Input: part model. Units: mm. Frame: model coordinates. A direction names the side the tool comes from. Give positions to 0.01 mm unless a question says otherwise; leave off trailing zeros. Write each loop counter-clockwise with the first axis right and the second up, starting at its lowest first coordinate (ties: lowest second). Pieces come first, ordered by that corner, then holes. Notation, with made-up numbers: (51.25, -33) -> (86.25, -33) arc R8 cw to (86.25, -18) -> close; hole circle Ø4 at (55, 80.25). An arc over 180 degrees is marked (long way). Return JSON: item names as keys, results as strings. Group by question number.
Item 1: Section B-B, the plane y = 1.25. Return loops of the section in (x, z), then the cut area to 3 significant figures.
Item 2: Mould query, pull axis X, two halves, no side actions, for faces 1 (the face through (-3.226, -11.456, -7.007)), 2 (the face through (10, -5, -0.5)), 3 (the face through (9.7, -0.7, -6.3)), 4 (the face through (0, 7.4, -7)). Classes: released by +X, released by -X, zero draft, split by the parting line, or undercut.
Item 3: Section A-A, the plane x = -8. Return loops of the section in (y, z).
Item 4: Section C-C, the plane z = -4.75. Return loops of the section in (x, y), then the cut area to 3 significant figures.
Item 5: Pin query (flat end, axial travel): P1, Ø2, axis at x = 4, y = 5, coming from the +Z side; P2, Ø1.5, axis at x = -10, z = -3.5, coming from the -Y side; P3, Ø4, axis at y = -8, z = -3, coming from the -X side. Return the tip coordinate at first contact, or that it passes through.
Item 6: Section D-D, the plane x = -3.5. Return loops of the section in (y, z).
Item 7: Line query: line 1 (Y direction, x = 13.5, z = -2.25); line 2 (Y direction, x = 12.5, z = -6.6); line 3 (Z direction, x = -15.5, y = -4.5). Output: solid intervals per line, ascending. Write a range as [from, to].
Item 8: Set-up query: faces 5 (the face through (-14, 2.7, -3)), 6 (the face through (4.786, -1.051, 2.632)), 7 (the face through (14, -2.7, -3)). Return all of +Z, -Z, +X, -X, +Y, -Y with unobstructed straight access to the full face (end or side cutting, diameter ignored); none if empty.
from build123d import *

# Parameters (mm, degrees)
P_IDAT_VYSUNUT_M1_DEPTH  = 1.4
P_IDAT_VYSUNUT_M2_DEPTH  = 2.5
SKICA3_R                 = 2.7
ODEBRAT_VYSUNUT_M1_DEPTH = 2.5
P_IDAT_VYSUNUT_M3_DEPTH  = 7.5
ODEBRAT_START            = -7.5
ODEBRAT_VYSUNUT_M2_DEPTH = 7.5
SKICA9_W                 = 31.786483692
SKICA9_H                 = 14.8
P_IDAT_VYSUNUT_M5_DEPTH  = 1
SKICA6_R                 = 3.25
ODEBRAT_VYSUNUT_M3_DEPTH = 1.2
SKICA7_R                 = 0.95
ODEBRAT_VYSUNUT_M5_DEPTH = 7
P_IDAT_VYSUNUT_M7_DEPTH  = 1


with BuildPart() as part:
    # Skica1 → Přidat vysunutím1 (new body)
    with BuildSketch(Plane.XY):
        with BuildLine():
            ThreePointArc((-17.587282337, 6.5), (-18.735542789, 0.736163289), (-18.043073463, -5.1))
            Line((-18.043073463, -5.1), (-15.043073463, -5.1))
            Line((-15.043073463, -5.1), (-15.043073463, -6.5))
            Line((-15.043073463, -6.5), (17.587282337, -6.5))
            ThreePointArc((17.587282337, -6.5), (18.735542789, -0.736163289), (18.043073463, 5.1))
            Line((18.043073463, 5.1), (15.043073463, 5.1))
            Line((15.043073463, 5.1), (15.043073463, 6.5))
            Line((15.043073463, 6.5), (-17.587282337, 6.5))
        make_face()
    extrude(amount=P_IDAT_VYSUNUT_M1_DEPTH)

    # Skica2 → Přidat vysunutím2 (add)
    with BuildSketch(Plane.XY.offset(1.4)):
        with BuildLine():
            ThreePointArc((-4.9, 0), (4.82555799, -0.850876071), (-4.604493842, 1.675898702))
            Line((-4.604493842, 1.675898702), (-6.577848346, 2.394141003))
            ThreePointArc((-6.577848346, 2.394141003), (-6.893654271, 1.215537244), (-7, 0))
            Line((-7, 0), (-4.9, 0))
        make_face()
    extrude(amount=P_IDAT_VYSUNUT_M2_DEPTH)

    # Skica3 → Odebrat vysunutím1 (cut)
    with BuildSketch(Plane.XY.offset(1.4)):
        with Locations((-12.5, 0)):
            Circle(SKICA3_R)
        with Locations((12.5, 0)):
            Circle(SKICA3_R)
    extrude(amount=-ODEBRAT_VYSUNUT_M1_DEPTH, mode=Mode.SUBTRACT)

    # Skica4 → Přidat vysunutím3 (add)
    with BuildSketch(Plane(origin=(0, 0, 0), x_dir=(-1, 0, 0), z_dir=(0, 0, -1))):
        with BuildLine():
            Line((14.493241846, 6.5), (-14.493241846, 6.5))
            ThreePointArc((-14.493241846, 6.5), (-15.192361337, 4.636401214), (-15.652924941, 2.7))
            Line((-15.652924941, 2.7), (-12.5, 2.7))
            ThreePointArc((-12.5, 2.7), (-10.590811691, 1.909188309), (-9.8, 0))
            ThreePointArc((-9.8, 0), (-10.590811691, -1.909188309), (-12.5, -2.7))
            Line((-12.5, -2.7), (-15.652924941, -2.7))
            ThreePointArc((-15.652924941, -2.7), (-15.192361337, -4.636401214), (-14.493241846, -6.5))
            Line((-14.493241846, -6.5), (14.493241846, -6.5))
            ThreePointArc((14.493241846, -6.5), (15.192361337, -4.636401214), (15.652924941, -2.7))
            Line((15.652924941, -2.7), (12.5, -2.7))
            ThreePointArc((12.5, -2.7), (9.8, 0), (12.5, 2.7))
            Line((12.5, 2.7), (15.652924941, 2.7))
            ThreePointArc((15.652924941, 2.7), (15.192361337, 4.636401214), (14.493241846, 6.5))
        make_face()
    extrude(amount=P_IDAT_VYSUNUT_M3_DEPTH)

    # Skica5 → Odebrat vysunutím2 (cut)
    with BuildSketch(Plane(origin=(0, 0, 0), x_dir=(-1, 0, 0), z_dir=(0, 0, -1)).offset(ODEBRAT_START)):
        with BuildLine():
            Line((15.043073463, -6.5), (15.043073463, -5.1))
            ThreePointArc((15.043073463, -5.1), (14.784738094, -5.80651175), (14.493241846, -6.5))
            Line((14.493241846, -6.5), (15.043073463, -6.5))
        make_face()
        with BuildLine():
            ThreePointArc((-15.043073463, 5.1), (-14.784738094, 5.80651175), (-14.493241846, 6.5))
            Line((-14.493241846, 6.5), (-15.043073463, 6.5))
            Line((-15.043073463, 6.5), (-15.043073463, 5.1))
        make_face()
    extrude(amount=ODEBRAT_VYSUNUT_M2_DEPTH, mode=Mode.SUBTRACT)

    # Skica9 → Přidat vysunutím5 (add)
    with BuildSketch(Plane(origin=(0, 0, -7.5), x_dir=(-1, 0, 0), z_dir=(0, 0, -1))):
        Rectangle(SKICA9_W, SKICA9_H)
    extrude(amount=-P_IDAT_VYSUNUT_M5_DEPTH)

    # Skica6 → Odebrat vysunutím3 (cut)
    with BuildSketch(Plane(origin=(0, 0, -7.5), x_dir=(-1, 0, 0), z_dir=(0, 0, -1))):
        with Locations((-12.5, 0)):
            Circle(SKICA6_R)
        with Locations((12.5, 0)):
            Circle(SKICA6_R)
    extrude(amount=-ODEBRAT_VYSUNUT_M3_DEPTH, mode=Mode.SUBTRACT)

    # Skica7 → Odebrat vysunutím5 (cut)
    with BuildSketch(Plane(origin=(0, 0, -7.5), x_dir=(-1, 0, 0), z_dir=(0, 0, -1))):
        with Locations((10.083296, 4.829031143)):
            Circle(SKICA7_R)
        with Locations((-10.083296, -4.829031143)):
            Circle(SKICA7_R)
    extrude(amount=-ODEBRAT_VYSUNUT_M5_DEPTH, mode=Mode.SUBTRACT)

    # Skica12 → Přidat vysunutím7 (add)
    with BuildSketch(Plane(origin=(0, 0, -7.5), x_dir=(-1, 0, 0), z_dir=(0, 0, -1))):
        Polygon((-5, -7.4), (-1.5, -15.4), (1.5, -15.4), (5, -7.4), align=None)
    extrude(amount=-P_IDAT_VYSUNUT_M7_DEPTH)


solid = part.part
Answer below:
{
 "1": {"outline": "(-18.71, 0) -> (-14.89, 0) -> (-14.89, 1.4) -> (-18.71, 1.4) -> close; (-15.89, -7.5) -> (-15.5, -7.5) -> (-15.5, -6.5) -> (-15.89, -6.5) -> close; (-10.11, -6.3) -> (-9.5, -6.3) -> (-9.5, -7.5) -> (9.5, -7.5) -> (9.5, -6.3) -> (10.11, -6.3) -> (10.11, 1.4) -> (4.74, 1.4) -> (4.74, 3.9) -> (-6.89, 3.9) -> (-6.89, 1.4) -> (-10.11, 1.4) -> close; (14.89, 0) -> (18.71, 0) -> (18.71, 1.4) -> (14.89, 1.4) -> close; (15.5, -7.5) -> (15.89, -7.5) -> (15.89, -6.5) -> (15.5, -6.5) -> close", "area": "219 mm2"},
 "2": {"face 1": "released by -X", "face 2": "undercut", "face 3": "undercut", "face 4": "zero draft"},
 "3": {"outline": "(-7.4, -7.5) -> (7.4, -7.5) -> (7.4, -6.5) -> (6.5, -6.5) -> (6.5, 1.4) -> (-6.5, 1.4) -> (-6.5, -6.5) -> (-7.4, -6.5) -> close"},
 "4": {"outline": "(-15.65, -2.7) arc R15.88 ccw to (-14.49, -6.5) -> (14.49, -6.5) arc R15.88 ccw to (15.65, -2.7) -> (12.5, -2.7) arc R2.7 cw to (12.5, 2.7) -> (15.65, 2.7) arc R15.88 ccw to (14.49, 6.5) -> (-14.49, 6.5) arc R15.88 ccw to (-15.65, 2.7) -> (-12.5, 2.7) arc R2.7 cw to (-12.5, -2.7) -> close; hole circle Ø1.9 at (-10.08, 4.83); hole circle Ø1.9 at (10.08, -4.83)", "area": "337 mm2"},
 "5": {"P1": "stops at z = 1.4", "P2": "stops at y = -6.5", "P3": "stops at x = -14.71"},
 "6": {"outline": "(-10.83, -7.5) -> (7.4, -7.5) -> (7.4, -6.5) -> (6.5, -6.5) -> (6.5, 1.4) -> (3.43, 1.4) -> (3.43, 3.9) -> (-3.43, 3.9) -> (-3.43, 1.4) -> (-6.5, 1.4) -> (-6.5, -6.5) -> (-10.83, -6.5) -> close"},
 "7": {"line 1": "y = [-6.5, -2.7], [2.7, 6.5]", "line 2": "y = [-7.4, -3.25], [3.25, 7.4]", "line 3": "z = [-7.5, -6.5], [0, 1.4]"},
 "8": {"face 5": "-X", "face 6": "+Z", "face 7": "+X"}
}
